from build123d import *

# Parameters (mm, degrees)
F1_DEPTH = 45.75
F0_W     = 92.649092
F0_H     = 18
F2_DEPTH = 45.75


with BuildPart() as f1:
    # F0 (on Front) → F1 (new body, symmetric)
    with BuildSketch(Plane.XZ):
        Polygon((26.753499, -34.5), (-0.395593, -34.5), (-0.395593, -48.93963), (-16.746501, -48.93963), (-16.746501, -66.93963), (125.007659, 0), (54.253499, 0), (54.253499, -17.25), (26.753499, -17.25), align=None)
    extrude(amount=F1_DEPTH, both=True)

    # F0 (on Front) → F2 (join, symmetric)
    with BuildSketch(Plane.XZ):
        Polygon((26.753499, -34.5), (-0.395593, -34.5), (-0.395593, -48.93963), (-16.746501, -48.93963), (-16.746501, -66.93963), (125.007659, 0), (54.253499, 0), (54.253499, -17.25), (26.753499, -17.25), align=None)
        with Locations((-63.071047, -57.93963)):
            Rectangle(F0_W, F0_H)
    extrude(amount=F2_DEPTH, both=True)


solid = f1.part
Design review of the part built by this model. Coordinates are the model's own, in mm. A direction names the side the tool comes from. Give positions to 0.01 mm unless a question says otherwise; leave off trailing zeros. Write each loop counter-clockwise with the first axis right and the second up, starting at its lowest first coordinate (ties: lowest second). Pieces come first, ordered by that corner, then holes. Notation, with made-up numbers: M 66,-34 L 123,-34 A28 cw 123,-6 Z; hole C 80.5,19.25 d11. An arc over 180 degrees is marked long. Answer as a JSON object with one key per item and string values. Group by question number.
1) We need section B-B (x = -42.5). Give the boundary of the cut face in (y, z), and give its area (3 significant figures).
2) Tool access review of faces 1 (the face through (7, -45.75, -41)), 2 (the face through (54.253, -1, -9)): name each direction out of +Z, -Z, +X, -X, +Y, -Y from which nothing blocks a thin tool from reaching the whole face with its end or side.
3) For line 1 along Z through (x, y) = (-63.5, -35); line 2 along Z through (x, y) = (74, 15); line 3 along X through (y, z) = (-1, -63), list the stretches that pass through material, from the lowest coordinate up.
4) Clearance check with flat-ended pins moving along their axes: pin 1 Ø14 at (y, z) = (-8, -24.5) entering from -X; pin 2 Ø8.5 at (y, z) = (22, -6.5) entering from -X; pin 3 Ø12 at (y, z) = (-30.5, -27.5) entering from +X. State where each tip first meets the part, or that it passes through.
5) We need section A-A (y = -31). Give the boundary of the cut face in (x, z).
6) We need section C-C (z = -13). Give the boundary of the cut face in (x, y), and give its area (3 significant figures).
Answer key:
{
 "1": {"outline": "M -45.75,-66.94 L 45.75,-66.94 L 45.75,-48.94 L -45.75,-48.94 Z", "area": "1,650 mm²"},
 "2": {"face 1": "+Z, -Z, +X, -X, -Y", "face 2": "+Z, -X, +Y, -Y"},
 "3": {"line 1": "z = -66.94 to -48.94", "line 2": "z = -24.09 to 0", "line 3": "x = -109.4 to -8.4"},
 "4": {"pin 1": "stops at x = 26.75", "pin 2": "stops at x = 54.25", "pin 3": "stops at x = 79.48"},
 "5": {"outline": "M -109.4,-66.94 L -16.75,-66.94 L 125.01,0 L 54.25,0 L 54.25,-17.25 L 26.75,-17.25 L 26.75,-34.5 L -0.4,-34.5 L -0.4,-48.94 L -109.4,-48.94 Z"},
 "6": {"outline": "M 54.25,-45.75 L 97.48,-45.75 L 97.48,45.75 L 54.25,45.75 Z", "area": "3,960 mm²"}
}
